from build123d import *

# Parameters (mm, degrees)
F1_DEPTH = 25.4
F2_R     = 48.434429
F3_DEPTH = 1.18585
F4_R     = 47.525627
F5_DEPTH = 63.5


with BuildPart() as f1:
    # F0 (on Front) → F1 (new body)
    with BuildSketch(Plane.XZ):
        Polygon((29.021849, 50.267316), (-29.021849, 50.267316), (-58.043697, 0), (-29.021849, -50.267316), (29.021849, -50.267316), (58.043697, 0), align=None)
    extrude(amount=F1_DEPTH)

    # F2 (on face) → F3 (join)
    with BuildSketch(Plane(origin=(0, 0, 0), x_dir=(-1, 0, 0), z_dir=(0, 1, 0))):
        Circle(F2_R)
    extrude(amount=-F3_DEPTH)

    # F4 (on face) → F5 (cut, symmetric)
    with BuildSketch(Plane(origin=(0, 0, 0), x_dir=(-1, 0, 0), z_dir=(0, 1, 0))):
        Circle(F4_R)
    extrude(amount=F5_DEPTH, both=True, mode=Mode.SUBTRACT)


solid = f1.part
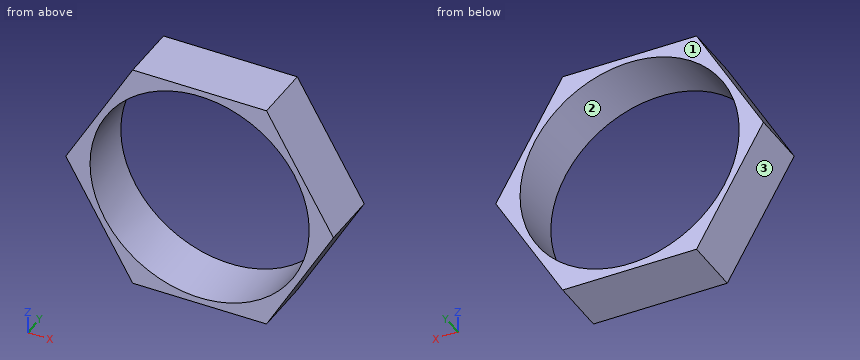
Check sheet for the modelled part. Datum: model origin and axes. Units: mm. Face numbers are marked on the shaded views. Round coordinates to 2 decimals unless told otherwise and drop trailing zeros. Loops run counter-clockwise (first coordinate to the right, second up) from the corner with the lowest first, then second, coordinate; pieces in that order, holes last. Notation, with made-up numbers: M -30.75,16 L 21.25,16 A24 cw 21.25,37 Z; hole C 8.5,-7.75 d2. An arc over 180 degrees is marked long. One line per item, written item: value.
(1) Sectioned sample at D-D, the plane x = -50. Record the cut outline in (y, z).
Computed values:
outline: M -25.4,-13.93 L 0,-13.93 L 0,13.93 L -25.4,13.93 Z
(2) Depth check by flat-ended pin: pin 1 Ø5 at (y, z) = (-6.5, -34.5) entering from +X; pin 2 Ø4 at (x, y) = (34, -17.5) entering from +Z; pin 3 Ø10 at (y, z) = (-15, -39) entering from +X. Enter the tip coordinate at first touch or a pass-through.
Computed values:
pin 1: stops at x = 39.57
pin 2: stops at z = 45.11
pin 3: stops at x = 38.41
(3) Thickness scan on line 1 (Z direction, x = 0, y = -19.75); line 2 (X direction, y = -6.75, z = -18); line 3 (Z direction, x = 22, y = -22). Record the ranges inside material, lowest first.
Computed values:
line 1: z = -50.27 to -47.53, 47.53 to 50.27
line 2: x = -47.65 to -43.99, 43.99 to 47.65
line 3: z = -50.27 to -42.13, 42.13 to 50.27
(4) Sectioned sample at B-B, the plane y = -17.25. Record the cut outline in (x, z), then the cut area to 3 significant figures.
Computed values:
outline: M -58.04,0 L -29.02,-50.27 L 29.02,-50.27 L 58.04,0 L 29.02,50.27 L -29.02,50.27 Z; hole C 0,0 d95.05
area: 1,660 mm^2
(5) Sectioned sample at A-A, the plane x = 0. Record the cut outline in (y, z), then the cut area to 3 significant figures.
Computed values:
outline: M -25.4,-50.27 L 0,-50.27 L 0,-47.53 L -25.4,-47.53 Z; M -25.4,47.53 L 0,47.53 L 0,50.27 L -25.4,50.27 Z
area: 139 mm^2
(6) Release check for a two-part mould opening along X. For the marked faces 1, 2 and 3 record: +X half, -X half, draft (parallel to the pull), parting line (faces both ways), or undercut.
Computed values:
face 1: draft
face 2: undercut
face 3: -X half
(7) Sectioned sample at C-C, the plane z = -34. Record the cut outline in (x, y), then the cut area to 3 significant figures.
Computed values:
outline: M -38.41,-25.4 L -33.21,-25.4 L -33.21,0 L -38.41,0 Z; M 33.21,-25.4 L 38.41,-25.4 L 38.41,0 L 33.21,0 Z
area: 265 mm^2
